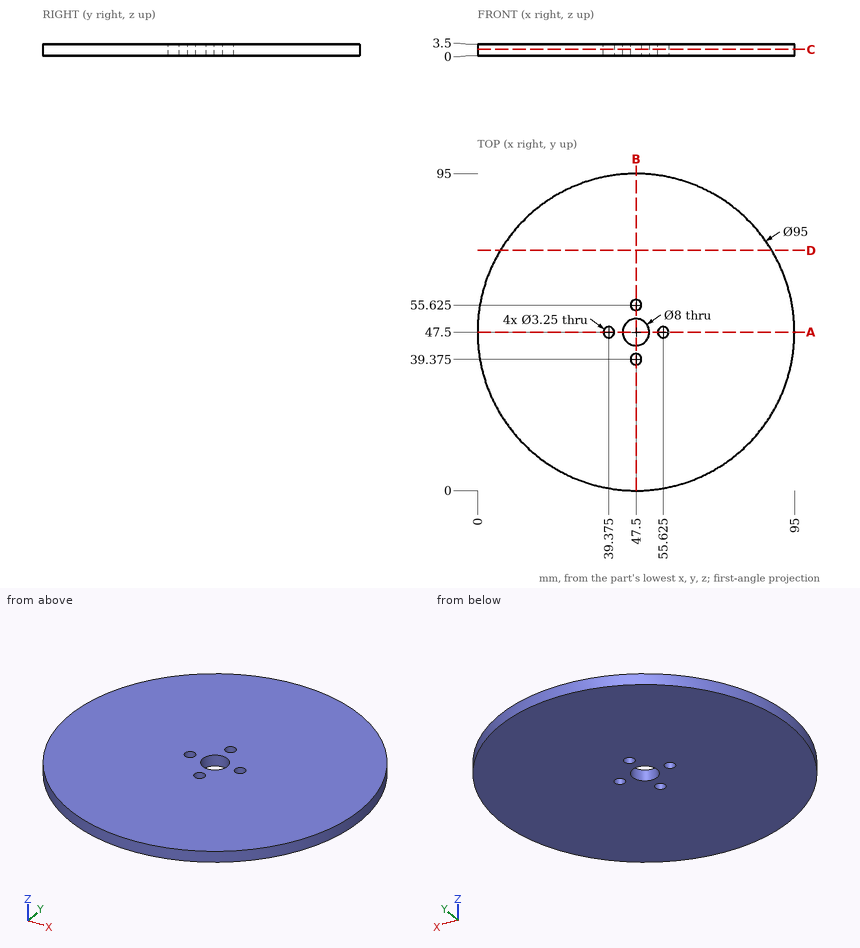
Geometry: see drawing. Coordinates: mm, zero at the bounding-box minimum. Round coordinates to 2 decimals unless told otherwise and drop trailing zeros. Loops run counter-clockwise (first coordinate to the right, second up) from the corner with the lowest first, then second, coordinate; pieces in that order, holes last. Notation, with made-up numbers: (46.5, -20) - (76.5, -20) arc R15 ccw to (76.5, -2) - close; hole circle Ø10 at (27, 82.25). An arc over 180 degrees is marked (long way). Use CSV: the item, a comma, the result in double quotes.
Q1. Section query A-A, the plane y = 47.5. Output: boundary loops of the cut face in (x, z).
Reported:
outline,"(0, 0) - (37.75, 0) - (37.75, 3.5) - (0, 3.5) - close; (41, 0) - (43.5, 0) - (43.5, 3.5) - (41, 3.5) - close; (51.5, 0) - (54, 0) - (54, 3.5) - (51.5, 3.5) - close; (57.25, 0) - (95, 0) - (95, 3.5) - (57.25, 3.5) - close"
Q2. Pin query (flat end, axial travel): pin 1 Ø10 at (x, y) = (62, 60.5) entering from -Z. Return the tip coordinate at first contact, or that it passes through.
Reported:
pin 1,"z = 0"
Q3. Section query D-D, the plane y = 72. Output: boundary loops of the cut face in (x, z).
Reported:
outline,"(6.81, 0) - (88.19, 0) - (88.19, 3.5) - (6.81, 3.5) - close"
Q4. Ray query, line 1 along Y through (x, z) = (47.5, 2.8); line 2 along Y through (x, z) = (56, 2.25); line 3 along Y through (x, z) = (38, 1.75). Return the intervals inside material, ascending.
Reported:
line 1,"0 to 37.75, 41 to 43.5, 51.5 to 54, 57.25 to 95"
line 2,"0.77 to 45.92, 49.08 to 94.23"
line 3,"0.96 to 46.63, 48.37 to 94.04"
Q5. Section query C-C, the plane z = 1.9. Output: boundary loops of the cut face in (x, y) (3 decimals).
Reported:
outline,"circle Ø95 at (47.5, 47.5); hole circle Ø3.25 at (39.375, 47.5); hole circle Ø8 at (47.5, 47.5); hole circle Ø3.25 at (47.5, 39.375); hole circle Ø3.25 at (47.5, 55.625); hole circle Ø3.25 at (55.625, 47.5)"
